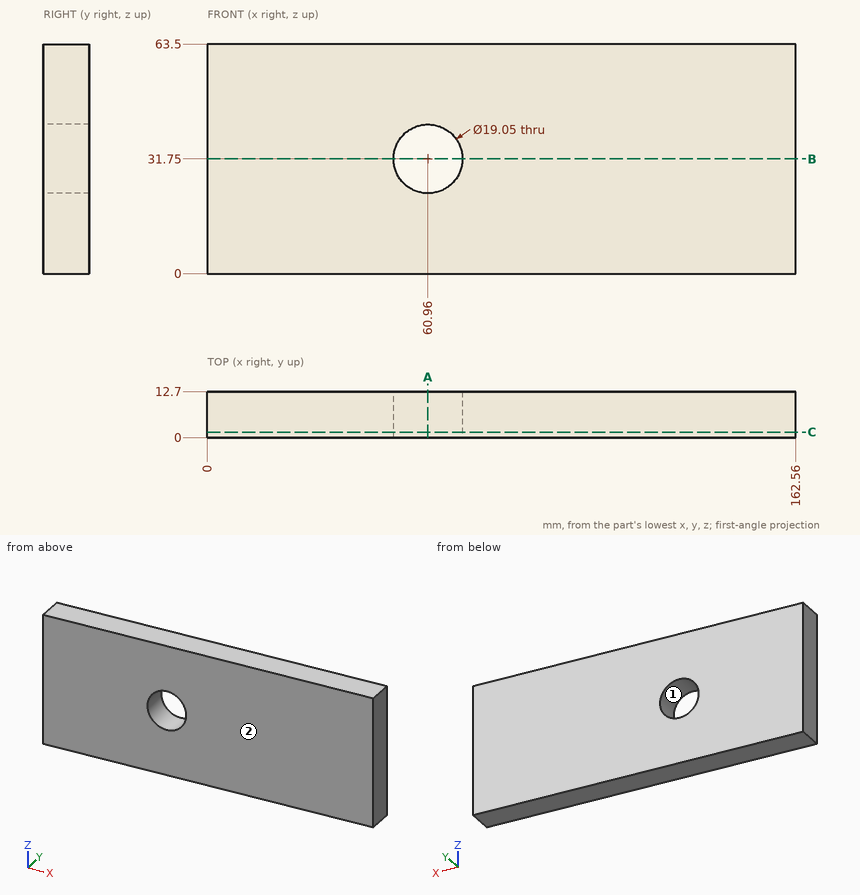
Design review of the part shown in the three views and the two pictorial views. Dimensions are in mm from the part's minimum x, y and z. Coordinates: 2 decimals unless noted, no trailing zeros. Loops run counter-clockwise (first coordinate to the right, second up) from the corner with the lowest first, then second, coordinate; pieces in that order, holes last. Notation, with made-up numbers: M 17,-32.5 L 37,-32.5 A20 ccw 37,-25.5 Z; hole C -19,-5.75 d3. An arc over 180 degrees is marked long. One line per question, with ' | ' between items.
(1) Wall thickness on probe 1 along Z at (x, y) = (60.96, 5.5) (3 decimals); probe 2 along X at (y, z) = (10.75, 35); probe 3 along X at (y, z) = (10, 30): over which ranges is each line inside the solid? List them lowest first.
Filled in:
probe 1: z = 0 to 22.225, 41.275 to 63.5 | probe 2: x = 0 to 52.01, 69.91 to 162.56 | probe 3: x = 0 to 51.6, 70.32 to 162.56
(2) Draft analysis for pull direction Z (two halves, no side actions). For the marked faces 1 and 2, state which applies: released by +Z, released by -Z, zero draft, split by the parting line, or undercut.
Filled in:
face 1: undercut | face 2: zero draft
(3) We need section B-B (z = 31.75). Give the boundary of the cut face in (x, y) (3 decimals).
Filled in:
outline: M 0,0 L 51.435,0 L 51.435,12.7 L 0,12.7 Z; M 70.485,0 L 162.56,0 L 162.56,12.7 L 70.485,12.7 Z
(4) We need section C-C (y = 1.5). Give the boundary of the cut face in (x, z) (3 decimals), and give its area (3 significant figures).
Filled in:
outline: M 0,0 L 162.56,0 L 162.56,63.5 L 0,63.5 Z; hole C 60.96,31.75 d19.05 | area: 10,000 mm^2
(5) We need section A-A (x = 60.96). Give the boundary of the cut face in (y, z) (3 decimals), and give its area (3 significant figures).
Filled in:
outline: M 0,0 L 12.7,0 L 12.7,22.225 L 0,22.225 Z; M 0,41.275 L 12.7,41.275 L 12.7,63.5 L 0,63.5 Z | area: 565 mm^2
